Part model, mm, in its own coordinate system. Round coordinates to 2 decimals unless told otherwise and drop trailing zeros. Order: outer loops, then holes, each group sorted by start corner. A loop starts at its lowest first (then second) coordinate and runs counter-clockwise, first axis right, second up. Notation, with made-up numbers: (-33.5, -4.5) -> (19.5, -4.5) arc R20 cw to (19.5, 9.5) -> close; hole circle Ø1 at (70, -29). An arc over 180 degrees is marked (long way). Return JSON: item names as keys, results as strings. Group by question number.
from build123d import *

# Parameters (mm, degrees)
SKIZZE2_R                       = 165
SKIZZE2_R_2                     = 136.5
AUFSATZ_LINEAR_AUSTRAGEN1_DEPTH = 3
DURCHGANGSLOCH_F_R_M101_D       = 11
KREISMUSTER1_COUNT              = 8


with BuildPart() as part:
    # Skizze2 → Aufsatz-Linear austragen1 (new body)
    with BuildSketch(Plane(origin=(0, 0, 0), x_dir=(0, 0, -1), z_dir=(1, 0, 0))):
        Circle(SKIZZE2_R)
        Circle(SKIZZE2_R_2, mode=Mode.SUBTRACT)
    extrude(amount=-AUFSATZ_LINEAR_AUSTRAGEN1_DEPTH)

    # Durchgangsloch für M101 (through all)
    with Locations(Plane(origin=(0, -26.503392929, -77.586576954), x_dir=(0, 0, -1), z_dir=(1, 0, 0))):
        with Locations((-77.586576954, 179.003392929)):
            durchgangsloch_f_r_m101 = Hole(DURCHGANGSLOCH_F_R_M101_D / 2)

    # Kreismuster1: Durchgangsloch für M101 ×8 about axis
    kreismuster1_axis = Axis((0, 0, 0), (1, 0, 0))
    for i in range(1, KREISMUSTER1_COUNT):
        add(durchgangsloch_f_r_m101.rotate(kreismuster1_axis, i * 360 / KREISMUSTER1_COUNT), mode=Mode.SUBTRACT)


solid = part.part
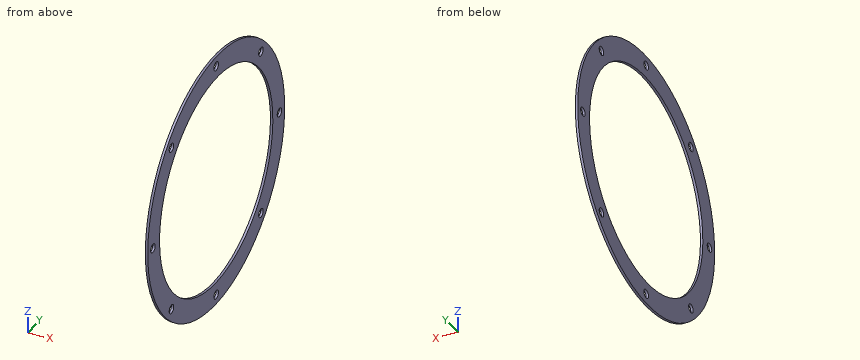
(1) Probe L1, parallel to Y at x = -0.9, z = 0; L2, parallel to Z at x = -1.3, y = -10; L3, parallel to Y at x = -1.25, z = 91. List the from-to ranges inside material, lowest first. Write a range as [from, to].
(2) Saw through at A-A, the plane z = 0. List the corners of the cut face in (x, y).
(3) Saw through at B-B, the plane y = 152.5. List the corners of the cut face in (x, z).
(4) Saw through at D-D, the plane z = -47. List the corners of the cut face in (x, y), and give its area (3 significant figures).
(5) Pin check, flat tips, straight feed: P1, Ø1, axis at x = -2, z = 3, coming from the +Y side; P2, Ø1, axis at x = -1, y = 16, coming from the +Z side; P3, Ø1.5, axis at x = -1.5, z = -73.5, coming from the +Y side; P4, Ø14.5, axis at y = 0, z = -152.5, coming from the -X side. Stop position of each tip, or through.
Results are:
{
 "1": {"L1": "y = [-165, -158], [-147, -136.5], [136.5, 147], [158, 165]", "L2": "z = [-164.7, -136.13], [136.13, 164.7]", "L3": "y = [-137.64, -101.74], [101.74, 137.64]"},
 "2": {"outline": "(-3, -165) -> (0, -165) -> (0, -158) -> (-3, -158) -> close; (-3, -147) -> (0, -147) -> (0, -136.5) -> (-3, -136.5) -> close; (-3, 136.5) -> (0, 136.5) -> (0, 147) -> (-3, 147) -> close; (-3, 158) -> (0, 158) -> (0, 165) -> (-3, 165) -> close"},
 "3": {"outline": "(-3, -63) -> (0, -63) -> (0, -5.5) -> (-3, -5.5) -> close; (-3, 5.5) -> (0, 5.5) -> (0, 63) -> (-3, 63) -> close"},
 "4": {"outline": "(-3, -158.16) -> (0, -158.16) -> (0, -128.15) -> (-3, -128.15) -> close; (-3, 128.15) -> (0, 128.15) -> (0, 158.16) -> (-3, 158.16) -> close", "area": "180 mm^2"},
 "5": {"P1": "stops at y = 164.98", "P2": "stops at z = 164.27", "P3": "stops at y = 148.1", "P4": "stops at x = -3"}
}
